from build123d import *

# Parameters (mm, degrees)
SKETCH1_R           = 95
SKETCH1_R_2         = 82.849042413
BOSS_EXTRUDE1_DEPTH = 2
SKETCH3_R           = 94.494442109
SKETCH3_R_2         = 91.333084699
BOSS_EXTRUDE2_DEPTH = 5
SKETCH4_W           = 62.439949526
SKETCH4_H           = 16.999481769
BOSS_EXTRUDE3_DEPTH = 20
SKETCH5_R           = 91.187715278
CUT_EXTRUDE1_DEPTH  = 20
SKETCH6_R           = 1.133326697
SKETCH6_R_2         = 0.88409454
SKETCH6_R_3         = 1.06382022
SKETCH6_R_4         = 1.11678576
SKETCH6_R_5         = 1.422635849
CUT_EXTRUDE2_DEPTH  = 25


with BuildPart() as part:
    # Sketch1 → Boss-Extrude1 (new body)
    with BuildSketch(Plane(origin=(0, 0, 0), x_dir=(1, 0, 0), z_dir=(0, 1, 0))):
        with Locations(Location((0, 0, 0), (0, 0, 270))):
            Circle(SKETCH1_R)
        with Locations(Location((0, 0, 0), (0, 0, 270))):
            Circle(SKETCH1_R_2, mode=Mode.SUBTRACT)
    extrude(amount=BOSS_EXTRUDE1_DEPTH)

    # Sketch3 → Boss-Extrude2 (add)
    with BuildSketch(Plane(origin=(0, 2, 0), x_dir=(1, 0, 0), z_dir=(0, 1, 0))):
        with Locations(Location((0, 0, 0), (0, 0, 270))):
            Circle(SKETCH3_R)
        with Locations(Location((0, 0, 0), (0, 0, 270))):
            Circle(SKETCH3_R_2, mode=Mode.SUBTRACT)
    extrude(amount=BOSS_EXTRUDE2_DEPTH)

    # Sketch4 → Boss-Extrude3 (add)
    with BuildSketch(Plane(origin=(0, 2, 0), x_dir=(1, 0, 0), z_dir=(0, 1, 0))):
        with Locations((-1.369214929, 92.645399109)):
            Rectangle(SKETCH4_W, SKETCH4_H)
    extrude(amount=BOSS_EXTRUDE3_DEPTH)

    # Sketch5 → Cut-Extrude1 (cut)
    with BuildSketch(Plane(origin=(0, 2, 0), x_dir=(1, 0, 0), z_dir=(0, 1, 0))):
        Circle(SKETCH5_R)
    extrude(amount=CUT_EXTRUDE1_DEPTH, mode=Mode.SUBTRACT)

    # Sketch6 → Cut-Extrude2 (cut)
    with BuildSketch(Plane(origin=(0, 0, -101.145139993), x_dir=(-1, 0, 0), z_dir=(0, 0, -1))):
        with Locations((22.112365303, 8.203766253)):
            Circle(SKETCH6_R)
        with Locations((4.179872068, 17.724091109)):
            Circle(SKETCH6_R_2)
        with Locations((-11.723213238, 5.51353779)):
            Circle(SKETCH6_R_3)
        with Locations((9.192330575, 9.220604642)):
            Circle(SKETCH6_R_4)
        with Locations((-19.090082193, 15.373412308)):
            Circle(SKETCH6_R_5)
    extrude(amount=-CUT_EXTRUDE2_DEPTH, mode=Mode.SUBTRACT)


solid = part.part
Could you check a few things on this model? Use its own coordinates, in mm. A direction names the side the tool comes from. Give positions to 0.01 mm unless a question says otherwise; leave off trailing zeros. Order: outer loops, then holes, each group sorted by start corner. A loop starts at its lowest first (then second) coordinate and runs counter-clockwise, first axis right, second up.
1. Will these pins go through, and if not, where does the flat tip stop? P1, Ø1.1, axis at x = -4.18, y = 17.72, coming from the -Z side; P2, Ø6, axis at x = -13, z = -96, coming from the -Y side; P3, Ø4.5, axis at y = 10, z = -90.5, coming from the +X side; P4, Ø10, axis at y = 2.5, z = 8.5, coming from the +X side.
2. Suppose I cut it at A-A (x = 0). List the corners of the cut face in (y, z) for me, plus the area to 3 significant figures.
3. Suppose I cut it at B-B (z = 0). List the corners of the cut face in (x, y) for me, plus the area to 3 significant figures.
4. I need wall thicknesses on L1, parallel to X at y = 5.65, z = 0; L2, parallel to X at y = 1.35, z = 0; L3, parallel to Z at x = 0, y = 5.1. Which ranges of each line are inside material? Lowest first, please.
5. For faces 1 (the cylindrical face through (-1.011, 11.86, -91.182)), 2 (the flat face through (78, 0, -29)), which set-ups out of +Z, -Z, +X, -X, +Y, -Y let a thin tool reach every point of the face, with its end or its side?
Solved:
1. P1: passes through
1. P2: stops at y = 0
1. P3: stops at x = 29.85
1. P4: stops at x = 94.93
2. outline: (0, -95) - (2, -95) - (2, -101.15) - (22, -101.15) - (22, -91.19) - (2, -91.19) - (2, -82.85) - (0, -82.85) - close; (0, 82.85) - (2, 82.85) - (2, 91.33) - (7, 91.33) - (7, 94.49) - (2, 94.49) - (2, 95) - (0, 95) - close
2. area: 264 mm2
3. outline: (-95, 0) - (-82.85, 0) - (-82.85, 2) - (-91.33, 2) - (-91.33, 7) - (-94.49, 7) - (-94.49, 2) - (-95, 2) - close; (82.85, 0) - (95, 0) - (95, 2) - (94.49, 2) - (94.49, 7) - (91.33, 7) - (91.33, 2) - (82.85, 2) - close
3. area: 80.2 mm2
4. L1: x = -94.49 to -91.33, 91.33 to 94.49
4. L2: x = -95 to -82.85, 82.85 to 95
4. L3: z = -101.15 to -91.19, 91.33 to 94.49
5. face 1: +Y
5. face 2: +Z, -Z, +X, -X, -Y
